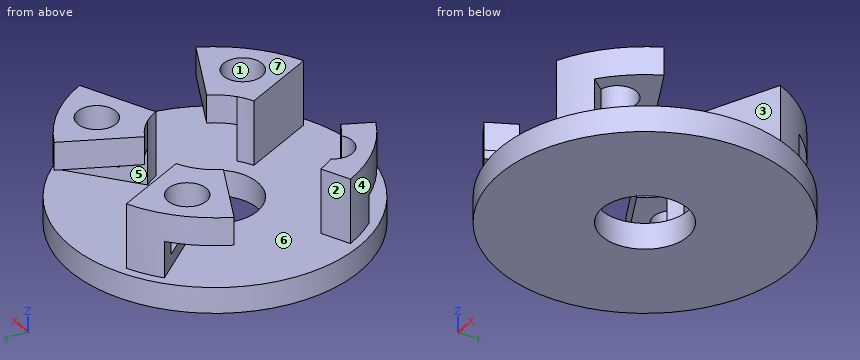
Autodesk Inventor part; units mm, degrees
ref_plane "YZ Plane" through (0, 0, 0) normal (1, 0, 0) x (0, 1, 0)
ref_plane "XZ Plane" through (0, 0, 0) normal (0, 1, 0) x (-1, 0, 0)
ref_plane "XY Plane" through (0, 0, 0) normal (0, 0, 1) x (1, 0, 0)
sketch "Sketch1" plane through (0, 0, 0) normal (0, 0, 1) x (1, 0, 0)
  circle A0 centre (0, 0) radius 34
  dimension "d0" = 68
extrude "Extrusion1" add sketch "Sketch1" along normal blind 6
sketch "Sketch2" plane through (0, 0, 6) normal (0, 0, 1) x (1, 0, 0)
  circle A0 centre (0, 0) radius 34
  circle A1 centre (0, 0) radius 34
  line L0 (0, 0) -> (30.6997, 14.6126) construction
  line L1 (0, 0) -> (25.8716, 22.0604) construction
  line L2 (25.8716, 22.0604) -> (10.653, 9.0837)
  line L3 (30.6997, 14.6126) -> (12.641, 6.017)
  arc A2 (30.6997, 14.6126) -> (25.8716, 22.0604) centre (0, 0) ccw
  arc A3 (12.641, 6.017) -> (10.653, 9.0837) centre (0, 0) ccw
  dimension "d3" = 15
  dimension "d4" = 20
extrude "Extrusion2" add sketch "Sketch2" along normal blind 15 contours L3 A3 L2 A0 picked at (22.8031, 15.025)
sketch "Sketch3" plane through (10.653, 9.0837, 21) normal (-0.6488347, 0.7609293, 0) x (0.7609293, 0.6488347, 0)
  line L0 (0, 15) -> (0, 0)
  line L1 (20, 0) -> (0, 0)
  line L2 (0, 0) -> (0, 6.5)
  line L3 (0, 6.5) -> (20, 6.5)
  line L4 (20, 6.5) -> (20, 0)
  line L5 (-14, 25.2) -> (-14, -4.2)
  line L6 (-48, 15) -> (20, 15)
  point P0 (-14, 21)
  point P1 (18.8415, 15)
  dimension "d7" = 6.5
  dimension "d26" = 8.5
revolve "Revolution1" add sketch "Sketch3" angle 25 about axis through (0, 0, 6) along (0, 0, 1)
sketch "Sketch4" plane through (0, 0, 21) normal (0, 0, 1) x (1, 0, 0)
  circle A0 centre (16.8356, 17.1044) radius 4.5
  arc A1 (12.641, 6.017) -> (5.816, 12.7348) centre (0, 0) ccw
  arc A2 (30.6997, 14.6126) -> (14.1245, 30.9273) centre (0, 0) ccw
  line L0 (12.641, 6.017) -> (30.6997, 14.6126)
  line L1 (5.816, 12.7348) -> (14.1245, 30.9273)
  arc A3 (21.6704, 10.3148) -> (9.9702, 21.831) centre (0, 0) ccw construction
  circle A4 centre (0, 0) radius 34 construction
  line L2 (23.8505, 24.2313) -> (19.6046, 19.9177) construction
  dimension "d12" = 9
extrude "Extrusion3" cut sketch "Sketch4" against normal blind 12 contours A0
pattern_circular "Circular Pattern2" count 4 over 360 about axis through (0, 0, 6) along (0, 0, 1) of "Revolution1", "Extrusion3", "Extrusion2"
sketch "Sketch5" plane through (0, 0, 0) normal (0, 0, -1) x (-1, 0, 0)
  circle A0 centre (0, 0) radius 10
  dimension "d23" = 20
extrude "Extrusion4" cut sketch "Sketch5" against normal blind 10
sketch "Sketch6" plane through (-14.1245, -30.9273, 14.5) normal (0, 0, -1) x (-0.9096266, 0.4154268, 0)
  line L0 (11.7881, 8.7204) -> (14.369, 3.1855)
  line L1 (0, 0) -> (0, 20)
  arc A0 (0, 0) -> (14.369, 3.1855) centre (0, 34) ccw
  arc A1 (0, 20) -> (5.9167, 21.3117) centre (0, 34) ccw
  arc A2 (0, 20) -> (5.9167, 21.3117) centre (0, 34) ccw
  arc A3 (0, 0) -> (14.369, 3.1855) centre (0, 34) ccw
  arc A4 (8.4204, 15.9424) -> (11.7881, 8.7204) centre (8.2085, 11.4474) ccw
  arc A5 (8.4204, 15.9424) -> (11.7881, 8.7204) centre (8.2085, 11.4474) ccw
  line L2 (14.369, 3.1855) -> (11.7881, 8.7204)
  line L3 (8.4204, 15.9424) -> (5.9167, 21.3117)
  point P0 (0, 34)
extrude "Extrusion5" add sketch "Sketch6" along normal blind 2
sketch "Sketch7" plane through (0, 0, 21) normal (0, 0, 1) x (0.7126851, -0.7014841, 0)
  line L0 (11.6287, -31.9495) -> (9.1517, -25.1441)
  line L1 (4.7883, -13.1557) -> (11.6287, -31.9495)
  line L2 (12.9105, -23.776) -> (15.3067, -30.3596)
  arc A0 (11.6287, -31.9495) -> (15.3067, -30.3596) centre (0, 0) ccw
  line L3 (12.9105, -23.776) -> (9.1517, -25.1441)
  arc A1 (-11.6287, -31.9495) -> (11.6287, -31.9495) centre (0, 0) ccw
  dimension "d29" = 4
extrude "Extrusion6" [suppressed]
sketch "Sketch8" plane through (-30.6997, -14.6126, 21) normal (0, 0, 1) x (0.9029321, 0.4297832, 0)
  circle A0 centre (34, 0) radius 34
  circle A1 centre (34, 0) radius 34
  circle A2 centre (34, 0) radius 10
  circle A3 centre (34, 0) radius 32
  dimension "d32" = 2
extrude "Extrusion7" cut sketch "Sketch8" against normal up to surface (15 mm away) contours A0
sketch "Sketch9" plane through (0, 0, 21) normal (0, 0, 1) x (0.7126851, -0.7014841, 0)
  point P0 (0, 0)
sketch "Sketch10" plane through (0, 0, 21) normal (0, 0, 1) x (0.7126851, -0.7014841, 0)
  line L0 (4.7883, -13.1557) -> (10.9208, -30.0046)
  line L1 (4.7883, -13.1557) -> (10.9446, -30.0702)
  line L2 (-4.7883, -13.1557) -> (-10.9446, -30.0702)
  line L3 (-4.7883, -13.1557) -> (-10.9446, -30.0702)
  arc A0 (-10.9446, -30.0702) -> (10.9446, -30.0702) centre (0, 0) ccw
  line L4 (7.8665, -21.6129) -> (10.9208, -30.0046)
  arc A1 (-8.5505, -23.4923) -> (8.5505, -23.4923) centre (0, 0) ccw
  line L5 (4.7883, -13.1557) -> (-4.7883, -13.1557)
  line L6 (10.9208, -30.0046) -> (15.734, -30.5587)
  line L7 (15.734, -30.5587) -> (12.8246, -22.565)
  line L8 (12.8246, -22.565) -> (9.1517, -25.1441)
  point P0 (0, 0)
  point P1 (14.6176, -28.4662)
  dimension "d36" = 7
extrude "Extrusion8" cut sketch "Sketch10" against normal up to surface (15 mm away) contours L0 A1 L2 L5
sketch "Sketch11" plane through (-11.1159, -24.3396, 21) normal (0, 0, 1) x (0.9096266, -0.4154268, 0)
  arc A0 (-20.5692, 2.2443) -> (4, -4.9913) centre (0, 26.7578) ccw
  point P0 (0, 26.7578)
properties part number "new male 4 bay con"
CAD build for the part. Positions are in the model's coordinates, mm. Face numbers are marked on the shaded views. A direction names the side the tool comes from. Round coordinates to 2 decimals unless told otherwise and drop trailing zeros. Write each loop counter-clockwise with the first axis right and the second up, starting at its lowest first coordinate (ties: lowest second). Pieces come first, ordered by that corner, then holes. Notation, with made-up numbers: M -25,25 L 28,25 A19 ccw 28,58 Z; hole C -25.5,34.25 d3. An arc over 180 degrees is marked long. Use a Markdown table: item, result. Add a question column.
1. 3-axis set-ups, long thin cutter, end or side, ignore diameter. For the marked faces 1, 2 and 3: which of +Z, -Z, +X, -X, +Y, -Y reach the whole face in a straight line?
2. Slice it at D-D on z = 19. Give the cut face in (x, y), then the cut area to 3 significant figures.
3. Drill centre lines: probe 1 along Z at (x, y) = (-17, -25); probe 2 along Y at (x, z) = (0, 3.4); probe 3 along Z at (x, y) = (6, 10.5). Where is each one in solid material? Low to high.
4. Pull direction Z, two halves, no side cores. Call the marked faces 4, 5, 6 and 7: released by +Z, released by -Z, zero draft, split by the parting line, or undercut.
5. Flat gauge pins, fed straight in: P1, Ø1.8, axis at x = -20, y = -16, coming from the +Z side; P2, Ø1.5, axis at x = -26, y = -23.5, coming from the +Z side; P3, Ø1, axis at x = 4, z = 4, coming from the +Y side; P4, Ø10, axis at x = -26.5, z = 14.5, coming from the +Y side. Where does each tip first touch, or does it go through?
6. Slice it at C-C on z = 7.5. Give the cut face in (x, y), then the cut area to 3 significant figures.
7. Slice it at A-A on y = 0. Give the cut face in (x, z), then the cut area to 3 significant figures.
Reply:
| question | item | result |
|---|---|---|
| 1 | face 1 | +Z |
| 1 | face 2 | +Z, -X |
| 1 | face 3 | +Z, +X |
| 2 | outline | M -29.11,13.29 L -12.73,5.82 A14 cw -9.08,10.65 A14 cw -6.02,12.64 L -13.75,28.89 A32 ccw Z; M -28.89,-13.75 A32 ccw -13.29,-29.11 L -10.39,-22.74 A25 cw -14.08,-20.66 A4.5 cw -20.43,-14.4 A25 cw -22.57,-10.74 Z; M 5.82,12.73 A14 cw 10.65,9.08 A14 cw 12.64,6.02 L 28.89,13.75 A32 ccw 13.29,29.11 Z; M 6.02,-12.64 L 13.75,-28.89 A32 ccw 29.11,-13.29 L 12.73,-5.82 A14 cw 9.08,-10.65 A14 cw Z; hole C -17.1,16.84 d9; hole C 16.84,17.1 d9; hole C 17.1,-16.84 d9 |
| 2 | area | 791 mm^2 |
| 3 | probe 1 | z = 0 to 6, 12.5 to 21 |
| 3 | probe 2 | y = -34 to -10, 10 to 34 |
| 3 | probe 3 | z = 0 to 6 |
| 4 | face 4 | zero draft |
| 4 | face 5 | undercut |
| 4 | face 6 | undercut |
| 4 | face 7 | released by +Z |
| 5 | P1 | stops at z = 9 |
| 5 | P2 | passes through |
| 5 | P3 | stops at y = 33.82 |
| 5 | P4 | stops at y = 23.7 |
| 6 | outline | M -28.89,-13.75 A32 ccw -24.35,-20.76 L -19.02,-16.22 A25 cw -22.57,-10.74 Z; M -20.76,24.35 L -9.08,10.65 A14 cw -6.02,12.64 L -13.75,28.89 A32 ccw Z; M 6.02,-12.64 L 13.75,-28.89 A32 ccw 20.76,-24.35 L 9.08,-10.65 A14 cw Z; M 10.65,9.08 A14 cw 12.64,6.02 L 28.89,13.75 A32 ccw 24.35,20.76 Z |
| 6 | area | 377 mm^2 |
| 7 | outline | M -34,0 L -10,0 L -10,6 L -34,6 Z; M 10,0 L 34,0 L 34,6 L 10,6 Z |
| 7 | area | 288 mm^2 |
